The figure shows three views and two pictorial views of one solid part (mm, origin at its lowest corner). Answer the questions. A direction names the side the tool comes from. Give positions to 0.01 mm unless a question says otherwise; leave off trailing zeros. Loops run counter-clockwise (first coordinate to the right, second up) from the corner with the lowest first, then second, coordinate; pieces in that order, holes last. Notation, with made-up numbers: (88, 41.5) - (106, 41.5) arc R21 ccw to (106, 79.5) - close; hole circle Ø11 at (-38.75, 78). An arc over 180 degrees is marked (long way). One line per question, with ' | ' between items.
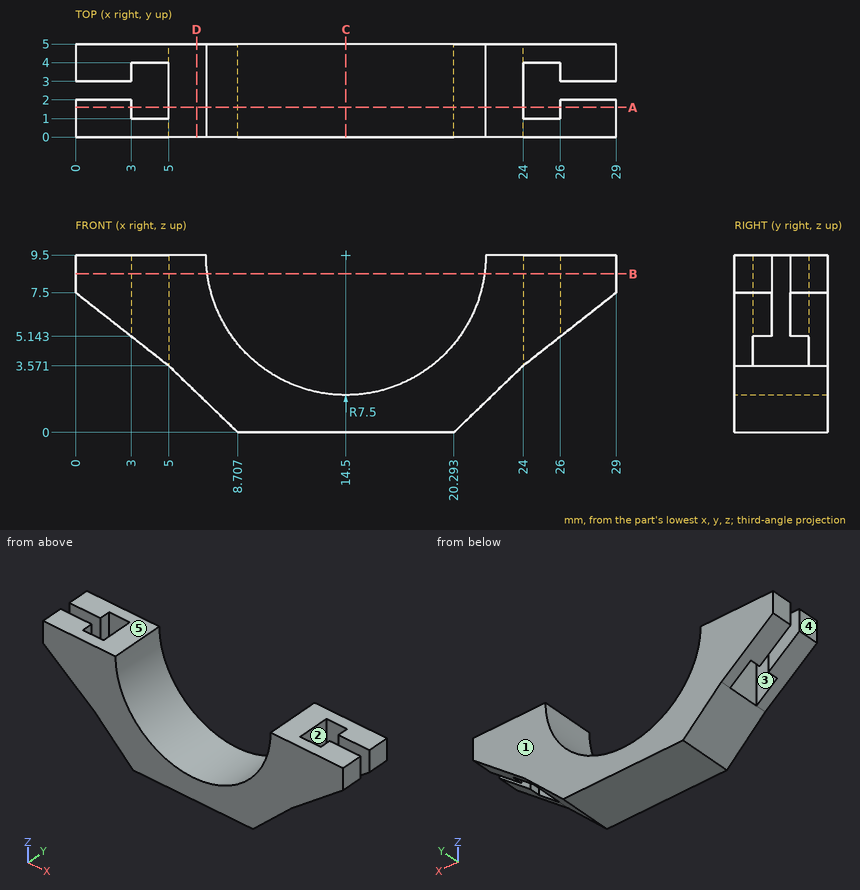
1. Flat-ended cylindrical pins translate along their axes: pin 1 (1 mm diameter, centred on x = 18, y = 4, fed in from -Z); pin 2 (0.5 mm diameter, centred on y = 3.5, z = 7, fed in from -X); pin 3 (1.5 mm diameter, centred on y = 0.5, z = 2.5, fed in from -X) (1 decimal); pin 4 (0.5 mm diameter, centred on y = 1.5, z = 6.5, fed in from +X) (1 decimal). Find the tip coordinate at first contact, or state that the pin passes through.
Evaluation:
pin 1: z = 0 | pin 2: x = 0.32 | pin 3: x = 5.3 | pin 4: x = 28
2. Determine the mould class of the marked faces 3, 4 and 5 for opening direction X: +X half, -X half, draft (parallel to the pull), parting line (faces both ways), or undercut.
Evaluation:
face 3: undercut | face 4: -X half | face 5: draft
3. Find section D-D on x = 6.5. Write down the section's boundary in (y, z).
Evaluation:
outline: (0, 2.13) - (5, 2.13) - (5, 9.5) - (0, 9.5) - close
4. Which of the six approach directions +Z, -Z, +X, -X, +Y, -Y give full straight-line access (tool end or side, diameter ignored) to the marked faces 1 and 2?
Evaluation:
face 1: +Z, -Z, +X, -X, +Y | face 2: +Z, -Z
5. Find section C-C on x = 14.5. Write down the section's boundary in (y, z).
Evaluation:
outline: (0, 0) - (5, 0) - (5, 2) - (0, 2) - close
6. Find section A-A on y = 1.6. Write down the section's boundary in (x, z).
Evaluation:
outline: (0, 7.5) - (3, 5.14) - (3, 9.5) - (0, 9.5) - close; (5, 3.57) - (8.71, 0) - (20.29, 0) - (24, 3.57) - (24, 9.5) - (22, 9.5) arc R7.5 cw to (7, 9.5) - (5, 9.5) - close; (26, 5.14) - (29, 7.5) - (29, 9.5) - (26, 9.5) - close
7. Consider L1, parallel to Y at x = 25.75, z = 5.75; L2, parallel to X at y = 1.4, z = 8.5; L3, parallel to X at y = 3.8, z = 7.25 (1 decimal). Determine where each line is inside the solid, lowest interval first.
Evaluation:
L1: 0 to 1, 4 to 5 | L2: 0 to 3, 5 to 7.07, 21.93 to 24, 26 to 29 | L3: 0.3 to 3, 5 to 7.3, 21.7 to 24, 26 to 28.7
8. Find section B-B on z = 8.5. Write down the section's boundary in (x, y).
Evaluation:
outline: (0, 0) - (7.07, 0) - (7.07, 5) - (0, 5) - (0, 3) - (3, 3) - (3, 4) - (5, 4) - (5, 1) - (3, 1) - (3, 2) - (0, 2) - close; (21.93, 0) - (29, 0) - (29, 2) - (26, 2) - (26, 1) - (24, 1) - (24, 4) - (26, 4) - (26, 3) - (29, 3) - (29, 5) - (21.93, 5) - close
